Job drawing, mm, ordinate dimensions from the low corner. One solid piece. A direction names the side the tool comes from. Give positions to 0.01 mm unless a question says otherwise; leave off trailing zeros. Loops run counter-clockwise (first coordinate to the right, second up) from the corner with the lowest first, then second, coordinate; pieces in that order, holes last. Notation, with made-up numbers: (-31.5, 83) -> (-19.5, 83) arc R34 cw to (-19.5, 116) -> close; hole circle Ø10 at (-26, 22.25). An arc over 180 degrees is marked (long way). Answer as a JSON object with one key per item and string values. Group by question number.
Q1. Drop flat-ended pins along their axis: pin 1 (3 mm diameter, centred on x = 13.175, y = 24.779, fed in from -Z); pin 2 (5.5 mm diameter, centred on x = 40.986, y = 5.221, fed in from -Z) (1 decimal). Give the stop position or say it passes through.
Q2. Wall check: probe 1 along X at (y, z) = (20.75, 4.7); probe 2 along X at (y, z) = (26.25, 4.2) (1 decimal); probe 3 along Y at (x, z) = (15, 0.45). Give the ranges that are in metal, low to high. Write a range as from..to.
Q3. Band-saw the part on B-B, the plane x = 4. Write the cut outline in (y, z).
Q4. Band-saw the part on A-A, the plane y = 20. Write the cut outline in (x, z).
Q5. Band-saw the part on C-C, the plane z = 1.05. Count the separate pieces of the cut face and the enclosed holes in it, plus the area to 3 significant figures.
Q6. Two-plate mould, pull along Y, no slides. Class the marked faces 1, 2, 3 and 4: pulls with the +Y half, pulls with the -Y half, needs draft (parallel to the pull), parting line crosses it, or undercut.
Q7. Band-saw the part on D-D, the plane y = 2.25. Write the cut outline in (x, z) (1 decimal), plus the area to 3 significant figures.
Q8. Tool access for the marked faces 5 and 6: list every direction of +Z, -Z, +X, -X, +Y, -Y with a clear straight run to the whole face (end or side of a thin tool).
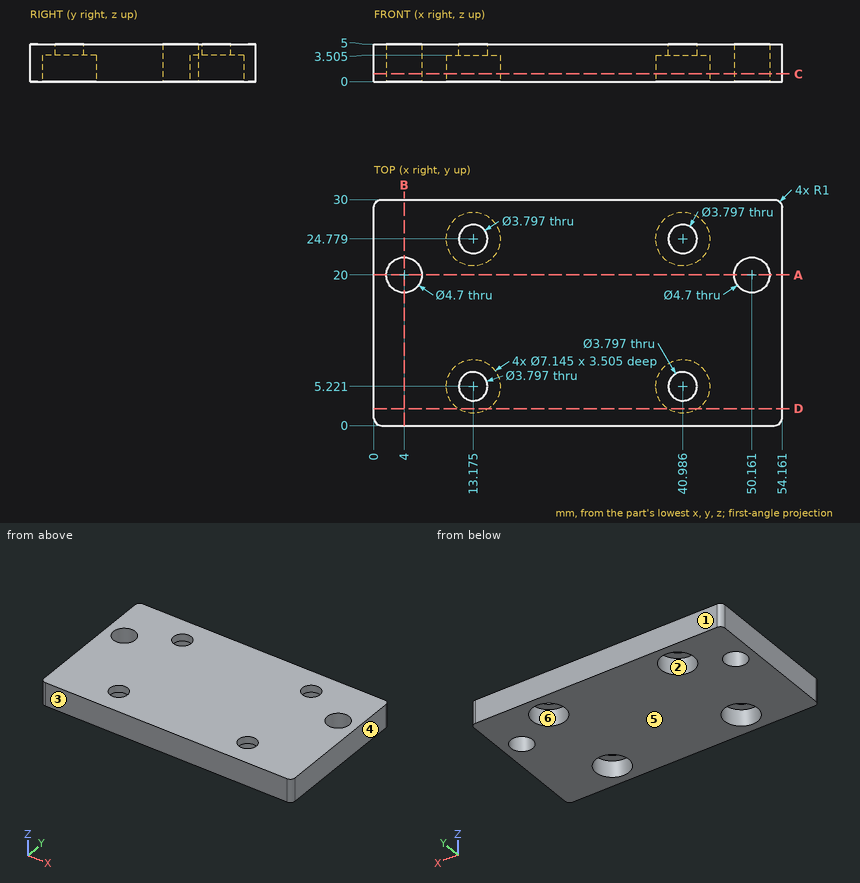
Worked answers:
{
 "1": {"pin 1": "through", "pin 2": "z = 3.5"},
 "2": {"probe 1": "0..1.77, 6.23..47.93, 52.39..54.16", "probe 2": "0..12, 14.4..39.8, 42.2..54.2", "probe 3": "0..2.15, 8.29..21.71, 27.85..30"},
 "3": {"outline": "(0, 0) -> (17.65, 0) -> (17.65, 5) -> (0, 5) -> close; (22.35, 0) -> (30, 0) -> (30, 5) -> (22.35, 5) -> close"},
 "4": {"outline": "(0, 0) -> (1.65, 0) -> (1.65, 5) -> (0, 5) -> close; (6.35, 0) -> (47.81, 0) -> (47.81, 5) -> (6.35, 5) -> close; (52.51, 0) -> (54.16, 0) -> (54.16, 5) -> (52.51, 5) -> close"},
 "5": {"separate pieces": "1", "enclosed holes": "6", "area": "1,430 mm2"},
 "6": {"face 1": "pulls with the +Y half", "face 2": "undercut", "face 3": "pulls with the -Y half", "face 4": "needs draft"},
 "7": {"outline": "(0, 0) -> (11.2, 0) -> (11.2, 3.5) -> (15.2, 3.5) -> (15.2, 0) -> (39, 0) -> (39, 3.5) -> (43, 3.5) -> (43, 0) -> (54.2, 0) -> (54.2, 5) -> (0, 5) -> close", "area": "243 mm2"},
 "8": {"face 5": "-Z, +X, -X, +Y, -Y", "face 6": "-Z"}
}
